The model under review builds one solid part; all positions refer to its coordinate system, in mm. Face numbers are marked on the shaded views. A direction names the side the tool comes from. Give positions to 0.01 mm unless a question says otherwise; leave off trailing zeros. Loops run counter-clockwise (first coordinate to the right, second up) from the corner with the lowest first, then second, coordinate; pieces in that order, holes last. Notation, with made-up numbers: M 15,-28.5 L 28,-28.5 A15 ccw 28,-11.5 Z; hole C 80,26 d5. An arc over 180 degrees is marked long. Put each result on its own line as item: value. Start each with the question number.
```python
from build123d import *

# Parameters (mm, degrees)
SZKIC1_R                    = 1.75
SZKIC1_R_2                  = 1
SZKIC1_W                    = 10
SZKIC1_H                    = 10
DODANIE_WYCI_GNI_CIE1_DEPTH = 2.5


with BuildPart() as part:
    # Szkic1 → Dodanie-wyciągnięcie1 (new body)
    with BuildSketch(Plane.XY):
        with BuildLine():
            Line((12.5, 0), (-12.5, 0))
            Line((-12.5, 0), (-12.5, 6.5))
            Line((-12.5, 6.5), (-9.25, 10.5))
            Line((-9.25, 10.5), (-9.25, 15.718810798))
            ThreePointArc((-9.25, 15.718810798), (0, 36), (9.25, 15.718810798))
            Line((9.25, 15.718810798), (9.25, 10.5))
            Line((9.25, 10.5), (12.5, 6.5))
            Line((12.5, 6.5), (12.5, 0))
        make_face()
        with Locations((0, 23.75)):
            Circle(SZKIC1_R, mode=Mode.SUBTRACT)
        with Locations((-5, 28)):
            Circle(SZKIC1_R_2, mode=Mode.SUBTRACT)
        with Locations((-5, 19.5)):
            Circle(SZKIC1_R_2, mode=Mode.SUBTRACT)
        with Locations(Location((5, 19.5, 0), (0, 0, 180))):
            Circle(SZKIC1_R_2, mode=Mode.SUBTRACT)
        with Locations(Location((5, 28, 0), (0, 0, 180))):
            Circle(SZKIC1_R_2, mode=Mode.SUBTRACT)
        with Locations((0, 10)):
            Rectangle(SZKIC1_W, SZKIC1_H, mode=Mode.SUBTRACT)
    extrude(amount=DODANIE_WYCI_GNI_CIE1_DEPTH)


solid = part.part
```
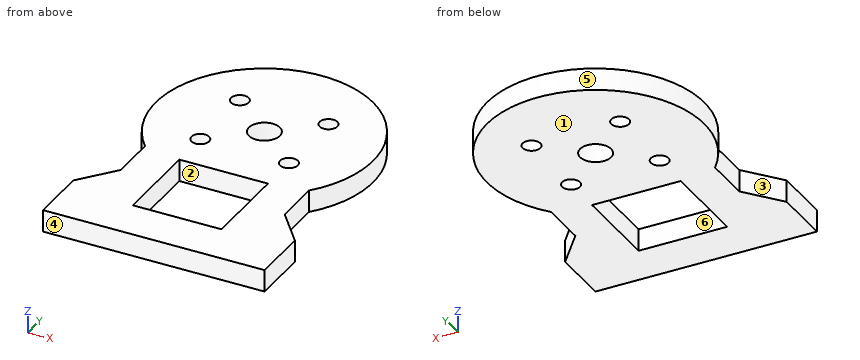
Item 1: Tool access review of the marked faces 1 and 2: name each direction out of +Z, -Z, +X, -X, +Y, -Y from which nothing blocks a thin tool from reaching the whole face with its end or side.
Item 2: Clearance check with flat-ended pins moving along their axes: pin 1 Ø2 at (x, y) = (-9, 7.5) entering from -Z; pin 2 Ø1.8 at (x, y) = (5, 28) entering from +Z. State where each tip first meets the part, or that it passes through.
Item 3: To check wall thickness, follow L1, parallel to Y at x = 0, z = 1.75; L2, parallel to X at y = 11, z = 0.45; L3, parallel to Y at x = -2.25, z = 1. State the ranges of each line that lie inside material, in increasing order. Write a range as [from, to].
Item 4: Consider section D-D, the plane y = 19.5. Write out the cut boundary in (x, z).
Item 5: Draft analysis for pull direction X (two halves, no side actions). For the marked faces 3, 4, 5 and 6, state which applies: +X half, -X half, draft (parallel to the pull), parting line (faces both ways), or undercut.
Item 6: Consider section B-B, the plane z = 0.7. Write out the cut boundary in (x, y).
Item 7: Consider section C-C, the plane y = 23.75. Write out the cut boundary in (x, z).
Item 8: Consider section A-A, the plane x = -2.25. Write out the cut boundary in (y, z).
Report:
1. face 1: -Z, +X, -X, +Y, -Y
1. face 2: +Z, -Z
2. pin 1: z = 0
2. pin 2: through
3. L1: [0, 5], [15, 22], [25.5, 36]
3. L2: [-9.25, -5], [5, 9.25]
3. L3: [0, 5], [15, 35.79]
4. outline: M -11.49,0 L -6,0 L -6,2.5 L -11.49,2.5 Z; M -4,0 L 4,0 L 4,2.5 L -4,2.5 Z; M 6,0 L 11.49,0 L 11.49,2.5 L 6,2.5 Z
5. face 3: -X half
5. face 4: draft
5. face 5: parting line
5. face 6: undercut
6. outline: M -12.5,0 L 12.5,0 L 12.5,6.5 L 9.25,10.5 L 9.25,15.72 A12.25 ccw long -9.25,15.72 L -9.25,10.5 L -12.5,6.5 Z; hole C -5,19.5 d2; hole C -5,28 d2; hole M -5,5 L 5,5 L 5,15 L -5,15 Z; hole C 0,23.75 d3.5; hole C 5,19.5 d2; hole C 5,28 d2
7. outline: M -12.25,0 L -1.75,0 L -1.75,2.5 L -12.25,2.5 Z; M 1.75,0 L 12.25,0 L 12.25,2.5 L 1.75,2.5 Z
8. outline: M 0,0 L 5,0 L 5,2.5 L 0,2.5 Z; M 15,0 L 35.79,0 L 35.79,2.5 L 15,2.5 Z
